Geometry: final body of the model. Coordinates: model frame, mm. Face numbers are marked on the shaded views. A direction names the side the tool comes from. Round coordinates to 2 decimals unless told otherwise and drop trailing zeros. Order: outer loops, then holes, each group sorted by start corner. A loop starts at its lowest first (then second) coordinate and runs counter-clockwise, first axis right, second up. Notation, with made-up numbers: (51.5, 73) -> (78.5, 73) arc R19 ccw to (78.5, 98) -> close; hole circle Ø3 at (-23, 0.5). An arc over 180 degrees is marked (long way). Put each result on its own line as item: value.
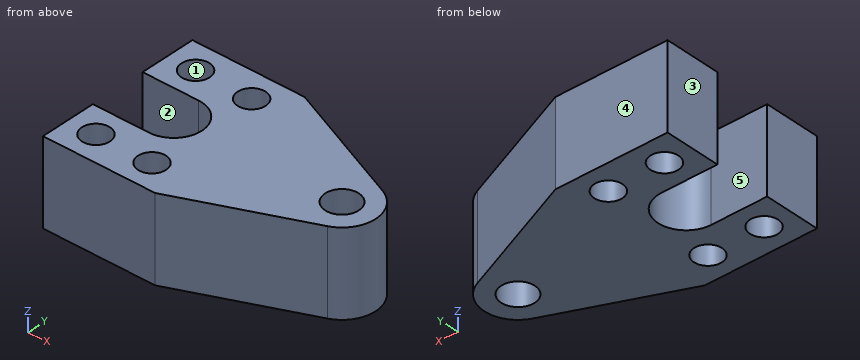
```python
from build123d import *

# Parameters (mm, degrees)
SKETCH1_R           = 5
SKETCH1_R_2         = 6
BOSS_EXTRUDE2_DEPTH = 15


with BuildPart() as part:
    # Sketch1 → Boss-Extrude2 (new, symmetric)
    with BuildSketch(Plane.XY):
        with BuildLine():
            Line((10, 10), (50, 10))
            Line((50, 10), (94.685564793, 28.952580276))
            ThreePointArc((94.685564793, 28.952580276), (102, 40), (94.685564793, 51.047419724))
            Line((94.685564793, 51.047419724), (50, 70))
            Line((50, 70), (10, 70))
            Line((10, 70), (10, 50))
            Line((10, 50), (30, 50))
            ThreePointArc((30, 50), (40, 40), (30, 30))
            Line((30, 30), (10, 30))
            Line((10, 30), (10, 10))
        make_face()
        with Locations((20, 60)):
            Circle(SKETCH1_R, mode=Mode.SUBTRACT)
        with Locations((40, 60)):
            Circle(SKETCH1_R, mode=Mode.SUBTRACT)
        with Locations((90, 40)):
            Circle(SKETCH1_R_2, mode=Mode.SUBTRACT)
        with Locations(Location((40, 20, 0), (0, 0, 180))):
            Circle(SKETCH1_R, mode=Mode.SUBTRACT)
        with Locations(Location((20, 20, 0), (0, 0, 180))):
            Circle(SKETCH1_R, mode=Mode.SUBTRACT)
    extrude(amount=BOSS_EXTRUDE2_DEPTH, both=True)


solid = part.part
```
1. Cut plane A-A on y = 40. Return loops of the section in (x, z), and give its area (3 significant figures).
Ans:
outline: (40, -15) -> (84, -15) -> (84, 15) -> (40, 15) -> close; (96, -15) -> (102, -15) -> (102, 15) -> (96, 15) -> close
area: 1,500 mm²
2. Cut plane C-C on z = -12.5. Return loops of the section in (x, y), and give its area (3 significant figures).
Ans:
outline: (10, 10) -> (50, 10) -> (94.69, 28.95) arc R12 ccw to (94.69, 51.05) -> (50, 70) -> (10, 70) -> (10, 50) -> (30, 50) arc R10 cw to (30, 30) -> (10, 30) -> close; hole circle Ø10 at (20, 20); hole circle Ø10 at (20, 60); hole circle Ø10 at (40, 20); hole circle Ø10 at (40, 60); hole circle Ø12 at (90, 40)
area: 3,370 mm²
3. Cut plane B-B on x = 20. Return loops of the section in (y, z), and give its area (3 significant figures).
Ans:
outline: (10, -15) -> (15, -15) -> (15, 15) -> (10, 15) -> close; (25, -15) -> (30, -15) -> (30, 15) -> (25, 15) -> close; (50, -15) -> (55, -15) -> (55, 15) -> (50, 15) -> close; (65, -15) -> (70, -15) -> (70, 15) -> (65, 15) -> close
area: 600 mm²
4. Contact query for flat-ended pins moving along their axis: P1, Ø11.5, axis at x = 20, y = 60, coming from the +Z side; P2, Ø12, axis at y = 24.5, z = 5, coming from the +X side. Output: stop coordinate, or through.
Ans:
P1: z = 15
P2: x = 97.33
5. Set-up query: the marked faces 4 and 5. Return all of +Z, -Z, +X, -X, +Y, -Y with unobstructed straight access to the full face (end or side cutting, diameter ignored); none if empty.
Ans:
face 4: +Z, -Z, +X, -X, +Y
face 5: +Z, -Z, -X
6. Draft query along X for the marked faces 1, 2 and 3. Return one class per face: +X half, -X half, draft (parallel to the pull), parting line (faces both ways), or undercut.
Ans:
face 1: undercut
face 2: draft
face 3: -X half
7. Material intervals for probe 1 along Y at (x, z) = (20, -5.5); probe 2 along Y at (x, z) = (36, -12.75); probe 3 along X at (y, z) = (20, -1.75), sorted ascending.
Ans:
probe 1: 10 to 15, 25 to 30, 50 to 55, 65 to 70
probe 2: 10 to 17, 23 to 32, 48 to 57, 63 to 70
probe 3: 10 to 15, 25 to 35, 45 to 73.58
8. Cut plane D-D on x = 33.5. Return loops of the section in (y, z), and give its area (3 significant figures).
Ans:
outline: (10, -15) -> (30.63, -15) -> (30.63, 15) -> (10, 15) -> close; (49.37, -15) -> (70, -15) -> (70, 15) -> (49.37, 15) -> close
area: 1,240 mm²
